```python
from build123d import *

# Parameters (mm, degrees)
F0_R      = 25
F1_DEPTH  = 55
F2_R      = 4
F14_T     = -2
F4_W      = 10
F4_H      = 5
F16_R     = 1
F3_R      = 23
F17_DEPTH = 50


with BuildPart() as f1:
    # F0 (on Top) → F1 (new body)
    with BuildSketch(Plane.XY):
        Circle(F0_R)
    extrude(amount=F1_DEPTH)

    # F2
    f2_edges = [f1.edges().sort_by_distance(p)[0] for p in [
        (-25, 0, 0),
    ]]
    fillet(f2_edges, radius=F2_R)

    # F14
    f14_openings = [f1.faces().sort_by_distance(p)[0] for p in [
        (0, 0, 55),
    ]]
    offset(amount=F14_T, openings=f14_openings)

    # F15: sweep along a path in F13
    with BuildLine(Plane.XZ) as f15_path:
        Line((0, 50), (33, 50))
        ThreePointArc((33, 50), (36.5355339059, 48.5355339059), (38, 45))
        Line((38, 45), (38, 5))
    # F4 (on Right) → F15 (sweep)
    with BuildSketch(Plane.YZ):
        with Locations((0, 50)):
            Rectangle(F4_W, F4_H)
    sweep(path=f15_path.line)

    # F16
    f16_edges = [f1.edges().sort_by_distance(p)[0] for p in [
        (40.5, -5, 25),
        (40.5, 5, 25),
        (35.5, -5, 25),
        (35.5, 5, 25),
    ]]
    fillet(f16_edges, radius=F16_R)

    # F3 (on face) → F17 (cut)
    with BuildSketch(Plane.XY.offset(55)):
        Circle(F3_R)
    extrude(amount=-F17_DEPTH, mode=Mode.SUBTRACT)


solid = f1.part
```
Here's how the part is built. I have some questions about the finished solid (model axes, mm). A direction names the side the tool comes from. Give positions to 0.01 mm unless a question says otherwise; leave off trailing zeros. Loops run counter-clockwise (first coordinate to the right, second up) from the corner with the lowest first, then second, coordinate; pieces in that order, holes last. Notation, with made-up numbers: M 25,56 L 31,56 A17 ccw 31,75 Z; hole C -6,-6.75 d9. An arc over 180 degrees is marked long. Put each result on its own line as item: value. Start each with the question number.
(1) If we mould it in two halves opening along X, with no side actions, what happens to faces 1 (the flat face through (29, 0, 47.5)), 2 (the flat face through (40.5, 0, 25)), 3 (the flat face through (38, 0, 5))? For each: +X half, -X half, draft (parallel to the pull), parting line (faces both ways), or undercut.
(2) For faces 4 (the flat face through (37, -5, 32)), 5 (the flat face through (0, 0, 2)), 6 (the flat face through (37, 5, 33)), which set-ups out of +Z, -Z, +X, -X, +Y, -Y let a thin tool reach every point of the face, with its end or its side?
(3) Will these pins go through, and if not, where does the flat tip stop? pin 1 Ø1.5 at (x, y) = (38, -0.5) entering from -Z; pin 2 Ø10 at (x, z) = (19, 29.5) entering from -Y; pin 3 Ø2 at (y, z) = (9.5, 6.5) entering from -X.
(4) I need wall thicknesses on line 1 along Y through (x, z) = (0, 26); line 2 along X through (y, z) = (6, 42); line 3 along X through (y, z) = (10.5, 45). Which ranges of each line are inside material? Lowest first, please. Write a range as [from, to].
(5) I want a section at C-C on x = 0. Please give me the cut outline in (y, z), then the cut area to 3 significant figures.
(6) I want a section at B-B on x = 29. Please give me the cut outline in (y, z).
(7) I want a section at A-A on z = 31. Please give me the cut outline in (x, y), then the cut area to 3 significant figures.
Answer block:
1. face 1: undercut
1. face 2: +X half
1. face 3: draft
2. face 4: +Z, -Z, +X, -Y
2. face 5: +Z
2. face 6: +Z, -Z, +X, +Y
3. pin 1: z = 5
3. pin 2: y = -20.71
3. pin 3: x = -23.51
4. line 1: [-25, -23], [23, 25]
4. line 2: [-24.27, -22.2], [22.2, 24.27]
4. line 3: [-22.69, -20.46], [20.46, 22.69]
5. outline: M -25,4 A4 ccw -21,0 L 21,0 A4 ccw 25,4 L 25,55 L 23,55 L 23,4 A2 cw 21,2 L -21,2 A2 cw -23,4 L -23,55 L -25,55 Z
5. area: 307 mm^2
6. outline: M -5,48.5 A1 ccw -4,47.5 L 4,47.5 A1 ccw 5,48.5 L 5,51.5 A1 ccw 4,52.5 L -4,52.5 A1 ccw -5,51.5 Z
7. outline: C 0,0 d50; M 35.5,-4 A1 ccw 36.5,-5 L 39.5,-5 A1 ccw 40.5,-4 L 40.5,4 A1 ccw 39.5,5 L 36.5,5 A1 ccw 35.5,4 Z; hole C 0,0 d46
7. area: 351 mm^2
